```python
from build123d import *

# Parameters (mm, degrees)
F0_R       = 120.65
F1_DEPTH   = 101.6
F2_SIZE2   = 19.05
F2_SIZE    = 25.4
F2_2_SIZE2 = 19.05
F2_2_SIZE  = 25.4
F3_R       = 12.7
F4_DEPTH   = 101.6


with BuildPart() as f1:
    # F0 (on Front) → F1 (new body)
    with BuildSketch(Plane.XZ):
        Circle(F0_R)
    extrude(amount=F1_DEPTH)

    # F2
    f2_edges = [f1.edges().sort_by_distance(p)[0] for p in [
        (-120.65, -101.6, 0),
    ]]
    f2_side = f1.faces().sort_by_distance((0, -101.6, 0))[0]
    chamfer(f2_edges, length=F2_SIZE, length2=F2_SIZE2, reference=f2_side)

    # F2#2
    f2_2_edges = [f1.edges().sort_by_distance(p)[0] for p in [
        (-120.65, 0, 0),
    ]]
    f2_2_side = f1.faces().sort_by_distance((0, 0, 0))[0]
    chamfer(f2_2_edges, length=F2_2_SIZE, length2=F2_2_SIZE2, reference=f2_2_side)

    # F3 (on face) → F4 (cut, through all)
    with BuildSketch(Plane.XZ.offset(101.6)):
        Circle(F3_R)
    extrude(amount=-F4_DEPTH, mode=Mode.SUBTRACT)


solid = f1.part
```
Geometry: final body of the model. Coordinates: model frame, mm. Coordinates: 2 decimals unless noted, no trailing zeros. Loops run counter-clockwise (first coordinate to the right, second up) from the corner with the lowest first, then second, coordinate; pieces in that order, holes last. Notation, with made-up numbers: (72.5, 13.25) -> (131.5, 13.25) arc R26 ccw to (131.5, 31.25) -> close; hole circle Ø4 at (37.25, -13.5). An arc over 180 degrees is marked (long way). Use a Markdown table: item, result. Add a question column.
(1) Mould query, pull axis X, two halves, no side actions, for faces 1 (the cylindrical face through (-120.533, -50.356, 5.305)), 2 (the cylindrical face through (-2.75, -51.51, -12.4)), 3 (the flat face through (-1, -101.6, -20)). Classes: pulls with the +X half, pulls with the -X half, needs draft (parallel to the pull), parting line crosses it, or undercut.
(2) Section query D-D, the plane y = -73. Return loops of the section in (x, z), plus the area to 3 significant figures.
(3) Pin query (flat end, axial travel): pin 1 Ø1 at (x, z) = (-85, 85.5) entering from -Y; pin 2 Ø5 at (x, z) = (-78.5, -83.5) entering from +Y; pin 3 Ø1.5 at (y, z) = (-76, 26.5) entering from -X; pin 4 Ø15 at (x, z) = (0, 0) entering from -Y. Return the tip coordinate at first contact, or that it passes through.
(4) Section query B-B, the plane x = 0. Return loops of the section in (y, z), plus the area to 3 significant figures.
(5) Section query C-C, the plane y = -89. Return loops of the section in (x, z).
(6) Line query: line 1 along Z through (x, y) = (0, -69); line 2 along Z through (x, y) = (2, -64); line 3 along X through (y, z) = (-7, 70). Output: solid intervals per line, ascending.
(7) Section query A-A, the plane z = 0. Return loops of the section in (x, y), plus the area to 3 significant figures.
Answer:
| question | item | result |
|---|---|---|
| 1 | face 1 | parting line crosses it |
| 1 | face 2 | undercut |
| 1 | face 3 | needs draft |
| 2 | outline | circle Ø241.3 at (0, 0); hole circle Ø25.4 at (0, 0) |
| 2 | area | 45,200 mm^2 |
| 3 | pin 1 | stops at y = -82.99 |
| 3 | pin 2 | stops at y = -12.64 |
| 3 | pin 3 | stops at x = -117.87 |
| 3 | pin 4 | passes through |
| 4 | outline | (-101.6, -95.25) -> (-82.55, -120.65) -> (-19.05, -120.65) -> (0, -95.25) -> (0, -12.7) -> (-101.6, -12.7) -> close; (-101.6, 12.7) -> (0, 12.7) -> (0, 95.25) -> (-19.05, 120.65) -> (-82.55, 120.65) -> (-101.6, 95.25) -> close |
| 4 | area | 21,000 mm^2 |
| 5 | outline | circle Ø224.1 at (0, 0); hole circle Ø25.4 at (0, 0) |
| 6 | line 1 | z = -120.65 to -12.7, 12.7 to 120.65 |
| 6 | line 2 | z = -120.63 to -12.54, 12.54 to 120.63 |
| 6 | line 3 | x = -77.7 to 77.7 |
| 7 | outline | (-120.65, -82.55) -> (-95.25, -101.6) -> (-12.7, -101.6) -> (-12.7, 0) -> (-95.25, 0) -> (-120.65, -19.05) -> close; (12.7, -101.6) -> (95.25, -101.6) -> (120.65, -82.55) -> (120.65, -19.05) -> (95.25, 0) -> (12.7, 0) -> close |
| 7 | area | 21,000 mm^2 |
